The model under review builds one solid part; all positions refer to its coordinate system, in mm. Face numbers are marked on the shaded views. Round coordinates to 2 decimals unless told otherwise and drop trailing zeros. Order: outer loops, then holes, each group sorted by start corner. A loop starts at its lowest first (then second) coordinate and runs counter-clockwise, first axis right, second up. Notation, with made-up numbers: M 34,22.25 L 85,22.25 A26 cw 85,50.25 Z; hole C 21,-36 d6. An arc over 180 degrees is marked long. Answer as a JSON object with one key per item and string values. Group by question number.
1. Add section C-C on y = -40. State the section outline as (x, z) points.
2. Add section B-B on z = -12. State the section outline as (x, y) points.
3. Add section D-D on y = -18.5. State the section outline as (x, z) points, and give its area (3 significant figures).
4. Add section A-A on x = -77.23. State the section outline as (y, z) points.
5. Clearance check with a flat-ended pin moving along its axis: P1, Ø12, axis at y = -69, z = -3.5, coming from the +X side. State where the tip first meets the part, or that it passes through.
6. Mouldability with a two-part tool opening along Y and no side actions: class the marked faces 1, 2, 3 and 4 as released by +Y, released by -Y, zero draft, split by the parting line, or undercut.
7. To check wall thickness, follow probe 1 along Y at (x, z) = (-77.23, -9.5); probe 2 along X at (y, z) = (-40.5, -17.25); probe 3 along Y at (x, z) = (-78.5, -0.75). State the ranges of each line that lie inside material, in increasing order. Write a range as [from, to].
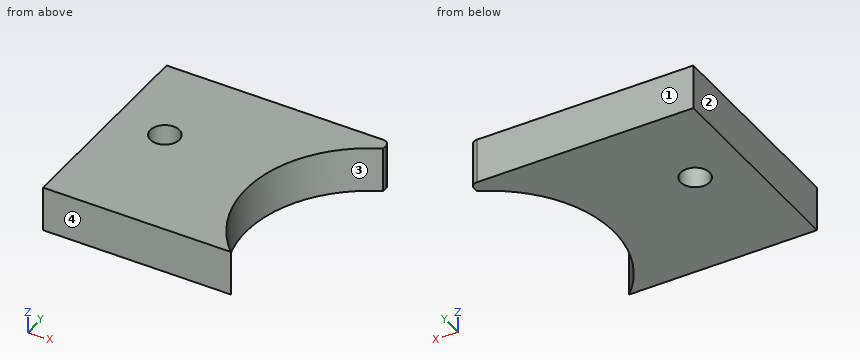
Solid Edge part; units mm, degrees
sketch "Sketch1" plane through (0, 0, 0) normal (0, 0, 1) x (1, 0, 0)
  line L0 (0, 0) -> (-100, 0)
  line L1 (-100, 0) -> (-100, -94)
  line L2 (-100, -94) -> (0, -94)
  line L3 (0, -94) -> (0, 0)
extrude "Protrusion1" add sketch "Sketch1" against normal blind 20.2
sketch "Sketch2" plane through (-50, -47, 0) normal (0, 0, 1) x (1, 0, 0)
  circle A0 centre (-27.23, 7) radius 6.5
  circle A1 centre (73, -8.1) radius 55
extrude "ExtrudedCutout_1" cut sketch "Sketch2" against normal blind 21
fillet "Round_1" radius 3 1 edges at (0, 0, -10.1)
Recorded:
{
 "1": {"outline": "M -100,-20.2 L -83.73,-20.2 L -83.73,0 L -100,0 Z; M -70.73,-20.2 L -29.89,-20.2 L -29.89,0 L -70.73,0 Z"},
 "2": {"outline": "M -100,-94 L -15.88,-94 A55 cw 0,-5.14 L 0,-3 A3 ccw -3,0 L -100,0 Z; hole C -77.23,-40 d13"},
 "3": {"outline": "M -100,-20.2 L -18.05,-20.2 L -18.05,0 L -100,0 Z", "area": "1,660 mm²"},
 "4": {"outline": "M -94,-20.2 L -46.5,-20.2 L -46.5,0 L -94,0 Z; M -33.5,-20.2 L 0,-20.2 L 0,0 L -33.5,0 Z"},
 "5": {"P1": "stops at x = -28.27"},
 "6": {"face 1": "released by +Y", "face 2": "zero draft", "face 3": "undercut", "face 4": "released by -Y"},
 "7": {"probe 1": "y = [-94, -46.5], [-33.5, 0]", "probe 2": "x = [-100, -83.71], [-70.75, -30.03]", "probe 3": "y = [-94, -46.37], [-33.63, 0]"}
}
